from build123d import *

# Parameters (mm, degrees)
F0_W     = 2340
F0_H     = 1260
F1_DEPTH = 27
F2_R     = 49.5
F3_DEPTH = 27.001


with BuildPart() as f1:
    # F0 (on Top) → F1 (new body)
    with BuildSketch(Plane.XY):
        with Locations((1170, 630)):
            Rectangle(F0_W, F0_H)
    extrude(amount=F1_DEPTH)

    # F2 (on face) → F3 (cut, through all)
    with BuildSketch(Plane.XY.offset(27)):
        with Locations((50, 1210)):
            Circle(F2_R)
        with Locations((1170, 1210)):
            Circle(F2_R)
        with Locations((2290, 1210)):
            Circle(F2_R)
        with Locations((2290, 50)):
            Circle(F2_R)
        with Locations((1170, 50)):
            Circle(F2_R)
        with Locations((50, 50)):
            Circle(F2_R)
    extrude(amount=-F3_DEPTH, mode=Mode.SUBTRACT)


solid = f1.part
Geometry: final body of the model. Coordinates: model frame, mm. Give positions to 0.01 mm unless a question says otherwise; leave off trailing zeros. Write each loop counter-clockwise with the first axis right and the second up, starting at its lowest first coordinate (ties: lowest second). Pieces come first, ordered by that corner, then holes. Notation, with made-up numbers: (70.25, 73) - (101.25, 73) arc R22 cw to (101.25, 95) - close; hole circle Ø8 at (24.25, 60). An arc over 180 degrees is marked (long way). Return JSON: item names as keys, results as strings. Group by question number.
1) Section C-C on x = 1170. Return the cut outline in (y, z).
2) Section B-B on z = 22.5. Return the cut outline in (x, y), plus the area to 3 significant figures.
3) Mould query, pull axis X, two halves, no side actions, for faces 1 (the flat face through (1154, 639, 0)), 2 (the cylindrical face through (2240.55, 52.18, 13.69)). Classes: released by +X, released by -X, zero draft, split by the parting line, or undercut.
4) Line query: line 1 (Y direction, x = 1170, z = 6.5); line 2 (X direction, y = 85.5, z = 2.25); line 3 (X direction, y = 82.5, z = 23). Output: solid intervals per line, ascending.
5) Section A-A on y = 50. Return the cut outline in (x, z), plus the area to 3 significant figures.
Filled in:
{
 "1": {"outline": "(0, 0) - (0.5, 0) - (0.5, 27) - (0, 27) - close; (99.5, 0) - (1160.5, 0) - (1160.5, 27) - (99.5, 27) - close; (1259.5, 0) - (1260, 0) - (1260, 27) - (1259.5, 27) - close"},
 "2": {"outline": "(0, 0) - (2340, 0) - (2340, 1260) - (0, 1260) - close; hole circle Ø99 at (50, 50); hole circle Ø99 at (50, 1210); hole circle Ø99 at (1170, 50); hole circle Ø99 at (1170, 1210); hole circle Ø99 at (2290, 50); hole circle Ø99 at (2290, 1210)", "area": "2,900,000 mm^2"},
 "3": {"face 1": "zero draft", "face 2": "undercut"},
 "4": {"line 1": "y = 0 to 0.5, 99.5 to 1160.5, 1259.5 to 1260", "line 2": "x = 0 to 15.5, 84.5 to 1135.5, 1204.5 to 2255.5, 2324.5 to 2340", "line 3": "x = 0 to 12.66, 87.34 to 1132.66, 1207.34 to 2252.66, 2327.34 to 2340"},
 "5": {"outline": "(0, 0) - (0.5, 0) - (0.5, 27) - (0, 27) - close; (99.5, 0) - (1120.5, 0) - (1120.5, 27) - (99.5, 27) - close; (1219.5, 0) - (2240.5, 0) - (2240.5, 27) - (1219.5, 27) - close; (2339.5, 0) - (2340, 0) - (2340, 27) - (2339.5, 27) - close", "area": "55,200 mm^2"}
}
